from build123d import *

# Parameters (mm, degrees)
SKETCH1_R           = 22
SKETCH1_R_2         = 7.93
BOSS_EXTRUDE1_DEPTH = 4
BOSS_EXTRUDE2_START = 11
SKETCH1_3_R         = 22
SKETCH1_3_R_2       = 20
BOSS_EXTRUDE2_DEPTH = 11
SKETCH1_4_R         = 19
CUT_EXTRUDE1_DEPTH  = 1.5
SKETCH3_R           = 11
SKETCH3_R_2         = 7.93
BOSS_EXTRUDE3_DEPTH = 1.5
CHAMFER1_SIZE       = 2.5


with BuildPart() as part:
    # Sketch1 → Boss-Extrude1 (new body)
    with BuildSketch(Plane(origin=(0, 0, 0), x_dir=(1, 0, 0), z_dir=(0, 1, 0))):
        with Locations(Location((0, 0, 0), (0, 0, 270))):
            Circle(SKETCH1_R)
        with Locations(Location((0, 0, 0), (0, 0, 270))):
            Circle(SKETCH1_R_2, mode=Mode.SUBTRACT)
    extrude(amount=-BOSS_EXTRUDE1_DEPTH)

    # Sketch1<3> → Boss-Extrude2 (add)
    with BuildSketch(Plane(origin=(0, 0, 0), x_dir=(1, 0, 0), z_dir=(0, 1, 0)).offset(BOSS_EXTRUDE2_START)):
        with Locations(Location((0, 0, 0), (0, 0, 270))):
            Circle(SKETCH1_3_R)
        with Locations(Location((0, 0, 0), (0, 0, 270))):
            Circle(SKETCH1_3_R_2, mode=Mode.SUBTRACT)
    extrude(amount=-BOSS_EXTRUDE2_DEPTH)

    # Sketch1<4> → Cut-Extrude1 (cut)
    with BuildSketch(Plane(origin=(0, 0, 0), x_dir=(1, 0, 0), z_dir=(0, 1, 0))):
        with Locations(Location((0, 0, 0), (0, 0, 270))):
            Circle(SKETCH1_4_R)
    extrude(amount=-CUT_EXTRUDE1_DEPTH, mode=Mode.SUBTRACT)

    # Sketch3 → Boss-Extrude3 (add)
    with BuildSketch(Plane.XZ.offset(4)):
        with Locations(Location((0, 0, 0), (0, 0, 90))):
            Circle(SKETCH3_R)
        with Locations(Location((0, 0, 0), (0, 0, 90))):
            Circle(SKETCH3_R_2, mode=Mode.SUBTRACT)
    extrude(amount=BOSS_EXTRUDE3_DEPTH)

    # Chamfer1
    # the kernel refuses this chamfer: 2.5 mm, written as the material it takes off along each edge
    with BuildSketch(Plane(origin=(0, -5.5, 0), x_dir=(0, 0, 1), z_dir=(1, 0, 0))) as chamfer1_piece_1_section:
        Polygon((11 - CHAMFER1_SIZE, 0), (11, -CHAMFER1_SIZE), (11, 0), align=None)
    chamfer1_piece_1 = revolve(axis=Axis((0, -5.5, 0), (0, -1, 0)), mode=Mode.PRIVATE)
    chamfer1_piece_1 = split(chamfer1_piece_1, bisect_by=Plane(origin=(0, -4, -9.254586784), z_dir=(0, -1, 0)), keep=Keep.TOP, mode=Mode.PRIVATE)
    add(chamfer1_piece_1, mode=Mode.SUBTRACT)


solid = part.part
Design review of the part built by this model. Coordinates are the model's own, in mm. A direction names the side the tool comes from. Round coordinates to 2 decimals unless told otherwise and drop trailing zeros. Loops run counter-clockwise (first coordinate to the right, second up) from the corner with the lowest first, then second, coordinate; pieces in that order, holes last. Notation, with made-up numbers: M 63,74.25 L 79,74.25 A20 cw 79,90.25 Z; hole C 3,89 d6. An arc over 180 degrees is marked long. Answer as a JSON object with one key per item and string values.
Item 1: We need section C-C on y = 2. Give the boundary of the cut face in (x, z), and give its area (3 significant figures).
Answer sheet:
{"outline": "C 0,0 d44; hole C 0,0 d40", "area": "264 mm^2"}
Item 2: We need section B-B on z = 0. Give the boundary of the cut face in (x, y).
Answer sheet:
{"outline": "M -22,-4 L -10,-4 L -8.5,-5.5 L -7.93,-5.5 L -7.93,-1.5 L -19,-1.5 L -19,0 L -20,0 L -20,11 L -22,11 Z; M 7.93,-5.5 L 8.5,-5.5 L 10,-4 L 22,-4 L 22,11 L 20,11 L 20,0 L 19,0 L 19,-1.5 L 7.93,-1.5 Z"}
Item 3: We need section A-A on x = 0. Give the boundary of the cut face in (y, z).
Answer sheet:
{"outline": "M -5.5,-8.5 L -4,-10 L -4,-22 L 11,-22 L 11,-20 L 0,-20 L 0,-19 L -1.5,-19 L -1.5,-7.93 L -5.5,-7.93 Z; M -5.5,7.93 L -1.5,7.93 L -1.5,19 L 0,19 L 0,20 L 11,20 L 11,22 L -4,22 L -4,10 L -5.5,8.5 Z"}
Item 4: We need section D-D on z = -14. Give the boundary of the cut face in (x, y), and give its area (3 significant figures).
Answer sheet:
{"outline": "M -16.97,-4 L 16.97,-4 L 16.97,11 L 14.28,11 L 14.28,0 L 12.85,0 L 12.85,-1.5 L -12.85,-1.5 L -12.85,0 L -14.28,0 L -14.28,11 L -16.97,11 Z", "area": "156 mm^2"}
Item 5: Clearance check with flat-ended pins moving along their axes: P1, Ø20, axis at x = -6.5, z = -3.5, coming from the +Y side; P2, Ø1.5, axis at x = 9, y = 6, coming from the +Z side; P3, Ø3, axis at x = 12, y = 1, coming from the +Z side; P4, Ø2, axis at x = 3.5, z = -8, coming from the -Y side. State where each tip first meets the part, or that it passes through.
Answer sheet:
{"P1": "stops at y = -1.5", "P2": "stops at z = 20.39", "P3": "stops at z = 19.33", "P4": "stops at y = -5.5"}
Item 6: Machinability: for faces 1 (the flat face through (0.3, -1.5, 8.2)), 2 (the flat face through (-8, -5.5, 2)), which of the approach directions +Z, -Z, +X, -X, +Y, -Y give a long, thin tool a straight path to every point of the face, cutting with its end or side? Answer none if there is none.
Answer sheet:
{"face 1": "+Y", "face 2": "+Z, -Z, +X, -X, -Y"}
Item 7: Wall thickness on L1, parallel to X at y = 10, z = 0; L2, parallel to Y at x = 2, z = 15; L3, parallel to Z at x = 11, y = -0.5: over which ranges is each line inside the solid? List them lowest first. Write a range as from..to.
Answer sheet:
{"L1": "x = -22..-20, 20..22", "L2": "y = -4..-1.5", "L3": "z = -19.05..-15.49, 15.49..19.05"}
Item 8: The part is to be moulded in two halves that separate along X. For faces 3 (the cylindrical face through (-19.524, 5.577, -4.336)), 4 (the cylindrical face through (-21.477, 3.605, -4.769)), 5 (the flat face through (-9, -4, 5)), say which applies: pulls with the +X half, pulls with the -X half, needs draft (parallel to the pull), parting line crosses it, or undercut.
Answer sheet:
{"face 3": "undercut", "face 4": "parting line crosses it", "face 5": "needs draft"}
